from build123d import *

# Parameters (mm, degrees)
SKETCH_1_R      = 2.5
EXTRUDE_1_DEPTH = 10
EXTRUDE_2_DEPTH = 90
SKETCH_3_R      = 2.5
EXTRUDE_3_DEPTH = 10


with BuildPart() as part:
    # 草图1 → 凸台-拉伸1 (new body)
    with BuildSketch(Plane.XY):
        Circle(SKETCH_1_R)
    extrude(amount=EXTRUDE_1_DEPTH)

    # 草图2 → 凸台-拉伸2 (add)
    with BuildSketch(Plane.XY.offset(10)):
        Polygon((3.549191068, -0.056914546), (1.823884976, 3.045232355), (-1.725306092, 3.1021469), (-3.549191068, 0.056914546), (-1.823884976, -3.045232355), (1.725306092, -3.1021469), align=None)
    extrude(amount=EXTRUDE_2_DEPTH)

    # 草图3 → 凸台-拉伸3 (add)
    with BuildSketch(Plane.XY.offset(100)):
        Circle(SKETCH_3_R)
    extrude(amount=EXTRUDE_3_DEPTH)


solid = part.part
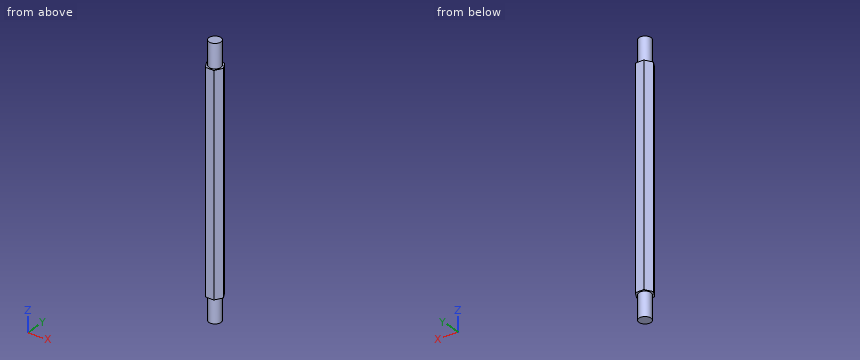
Verification items for the finished model (mm, model axes). Round coordinates to 2 decimals unless told otherwise and drop trailing zeros. Loops run counter-clockwise (first coordinate to the right, second up) from the corner with the lowest first, then second, coordinate; pieces in that order, holes last. Notation, with made-up numbers: (76, 42.25) - (85, 42.25) arc R37 ccw to (85, 79.25) - close; hole circle Ø4 at (84, 0.5). An arc over 180 degrees is marked (long way). Use one line per item in the form item = value.
1. Section check C-C on z = 76. Record the cut outline in (x, y), and give its area (3 significant figures).
A:
outline = (-3.55, 0.06) - (-1.82, -3.05) - (1.73, -3.1) - (3.55, -0.06) - (1.82, 3.05) - (-1.73, 3.1) - close
area = 32.7 mm²
2. Section check B-B on y = -1.25. Record the cut outline in (x, z), and give its area (3 significant figures).
A:
outline = (-2.82, 10) - (-2.17, 10) - (-2.17, 0) - (2.17, 0) - (2.17, 10) - (2.83, 10) - (2.83, 100) - (2.17, 100) - (2.17, 110) - (-2.17, 110) - (-2.17, 100) - (-2.82, 100) - close
area = 596 mm²
3. Gauge pin test, flat ends, axial feed: pin 1 Ø1 at (x, z) = (-0.5, 70.5) entering from +Y; pin 2 Ø1.5 at (y, z) = (1, 77.5) entering from -X; pin 3 Ø1 at (x, z) = (1, 23) entering from -Y. Record the tip position at first contact, or that the pin passes through.
A:
pin_1 = 3.09
pin_2 = -3.43
pin_3 = -3.1
4. Section check D-D on z = 102.5. Record the cut outline in (x, y), and give its area (3 significant figures).
A:
outline = circle Ø5 at (0, 0)
area = 19.6 mm²
5. Section check A-A on x = 0. Record the cut outline in (y, z), and give its area (3 significant figures).
A:
outline = (-3.07, 10) - (-2.5, 10) - (-2.5, 0) - (2.5, 0) - (2.5, 10) - (3.07, 10) - (3.07, 100) - (2.5, 100) - (2.5, 110) - (-2.5, 110) - (-2.5, 100) - (-3.07, 100) - close
area = 653 mm²
6. Scan lines: probe 1 along Y at (x, z) = (-1, 11); probe 2 along Z at (x, y) = (-1.75, -2); probe 3 along Y at (x, z) = (-2.5, 38). Record each from-to range of solid material in increasing order.
A:
probe_1 = -3.06 to 3.09
probe_2 = 10 to 100
probe_3 = -1.83 to 1.81
